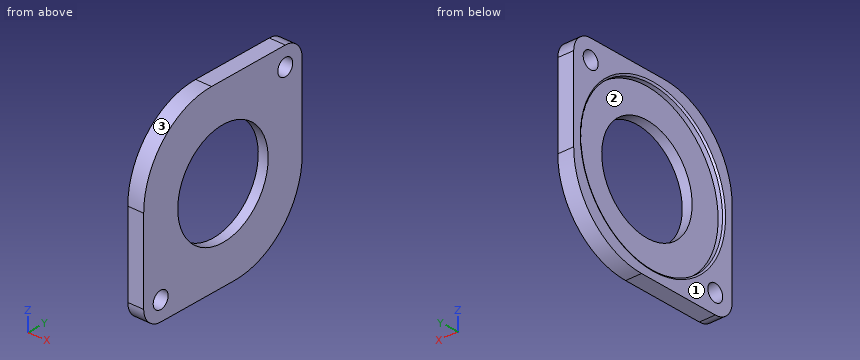
from build123d import *

# Parameters (mm, degrees)
SKETCH1_R             = 12.7
BOSS_EXTRUDE1_DEPTH   = 3.96875
SKETCH2_R             = 19.99742
CUT_EXTRUDE1_DEPTH    = 1.50114
F_8_CLEARANCE_HOLE1_D = 4.191
FILLET1_R             = 0.396875


with BuildPart() as part:
    # Sketch1 → Boss-Extrude1 (new body)
    with BuildSketch(Plane(origin=(0, 0, 0), x_dir=(0, 0, -1), z_dir=(1, 0, 0))):
        with BuildLine():
            Line((-17.5, 22.2625), (3.2125, 22.2625))
            ThreePointArc((3.2125, 22.2625), (16.682884182, 16.682884182), (22.2625, 3.2125))
            Line((22.2625, 3.2125), (22.2625, -17.5))
            ThreePointArc((22.2625, -17.5), (20.867596045, -20.867596045), (17.5, -22.2625))
            Line((17.5, -22.2625), (-3.2125, -22.2625))
            ThreePointArc((-3.2125, -22.2625), (-16.682884182, -16.682884182), (-22.2625, -3.2125))
            Line((-22.2625, -3.2125), (-22.2625, 17.5))
            ThreePointArc((-22.2625, 17.5), (-20.867596045, 20.867596045), (-17.5, 22.2625))
        make_face()
        Circle(SKETCH1_R, mode=Mode.SUBTRACT)
    extrude(amount=BOSS_EXTRUDE1_DEPTH)

    # Sketch2 → Cut-Extrude1 (cut)
    with BuildSketch(Plane.ZY):
        Circle(SKETCH2_R)
    extrude(amount=-CUT_EXTRUDE1_DEPTH, mode=Mode.SUBTRACT)

    # #8 Clearance Hole1 (through all)
    with Locations(Plane(origin=(3.96875, 0, 0), x_dir=(0, 0, -1), z_dir=(1, 0, 0))):
        with Locations((-17.5, 17.5), (17.5, -17.5)):
            Hole(F_8_CLEARANCE_HOLE1_D / 2)

    # Fillet1
    fillet1_edges = [part.edges().sort_by_distance(p)[0] for p in [
        (0, 0, -19.99742),
    ]]
    fillet(fillet1_edges, radius=FILLET1_R)


solid = part.part
Could you check a few things on this model? Use its own coordinates, in mm. Face numbers are marked on the shaded views. Coordinates: 2 decimals unless noted, no trailing zeros. Loops run counter-clockwise (first coordinate to the right, second up) from the corner with the lowest first, then second, coordinate; pieces in that order, holes last.
1. For P1, Ø6.5, axis at y = -17.5, z = -17.5, coming from the -X side; P2, Ø5, axis at y = -8.5, z = 13, coming from the -X side, each with a flat end and sliding along its axis, tell me the tip position at first contact or that it passes through.
2. I need wall thicknesses on L1, parallel to Y at x = 3.05, z = 0; L2, parallel to Y at x = 1.25, z = 17.5; L3, parallel to X at y = -14, z = -13.5. Which ranges of each line are inside material? Lowest first, please.
3. We'd pull the mould along Y, two halves only. Please class the marked faces 1, 2 and 3: released by +Y, released by -Y, zero draft, split by the parting line, or undercut.
4. Imagine slicing it at A-A (x = 2.45). Give the number of separate pieces and of enclosed holes in the cut face, and give its area (3 significant figures).
5. Imagine slicing it at B-B (z = 0). Please give me the cut outline in (x, y).
Computed values:
1. P1: stops at x = 0
1. P2: stops at x = 1.5
2. L1: y = -22.26 to -12.7, 12.7 to 22.26
2. L2: y = -15.81 to -9.68, 9.68 to 15.4, 19.6 to 22.26
2. L3: x = 1.5 to 3.97
3. face 1: zero draft
3. face 2: undercut
3. face 3: released by -Y
4. separate pieces: 1
4. enclosed holes: 3
4. area: 1,280 mm2
5. outline: (0, -22.26) - (3.97, -22.26) - (3.97, -12.7) - (1.5, -12.7) - (1.5, -20) - (0.4, -20) arc R0.4 ccw to (0, -20.39) - close; (0, 20.39) arc R0.4 ccw to (0.4, 20) - (1.5, 20) - (1.5, 12.7) - (3.97, 12.7) - (3.97, 22.26) - (0, 22.26) - close
